Read the model definition and answer for the solid it produces. Units are mm, in the model's axes. A direction names the side the tool comes from. Round coordinates to 2 decimals unless told otherwise and drop trailing zeros. Write each loop counter-clockwise with the first axis right and the second up, starting at its lowest first coordinate (ties: lowest second). Pieces come first, ordered by that corner, then holes.
from build123d import *

# Parameters (mm, degrees)
SKETCH034_R     = 3.75
POCKET013_DEPTH = 9.70192
CHAMFER013_SIZE = 0.4
CHAMFER014_SIZE = 0.1


with BuildPart() as pocket013:
    # Sketch035 → Revolution005 (revolve)
    with BuildSketch(Plane.XZ):
        Polygon((0, 0.29908), (2.75, 1.3), (2.75, 10), (0, 10), align=None)
    revolve(axis=Axis((0, 0, 0), (0, 0, 1)))

    # Sketch034 (on Face3 of Revolution005) → Pocket013 (cut, through all)
    with BuildSketch(Plane(origin=(0, 0, 10), x_dir=(-1, 0, 0), z_dir=(0, 0, 1))):
        Circle(SKETCH034_R)
        Polygon((-0.721688, 1.25), (0.721688, 1.25), (1.443376, 0), (0.721688, -1.25), (-0.721688, -1.25), (-1.443376, 0), align=None, mode=Mode.SUBTRACT)
    extrude(amount=-POCKET013_DEPTH, mode=Mode.SUBTRACT)


with BuildPart() as chamfer014:
    # Sketch033 → Revolution004 (revolve)
    with BuildSketch(Plane.XZ):
        Polygon((1.45, 3), (2.75, 3), (2.75, 0), (1.5, 0), (1.5, -10), (0, -10), (0, 1.549999), align=None)
    revolve(axis=Axis((0, 0, 0), (0, 0, 1)))

    # Cut005: cut Pocket013
    add(pocket013.part, mode=Mode.SUBTRACT)

    # Chamfer013
    chamfer013_edges = [chamfer014.edges().sort_by_distance(p)[0] for p in [
        (-1.5, 0, -10),
    ]]
    chamfer(chamfer013_edges, length=CHAMFER013_SIZE)

    # Chamfer014
    chamfer014_edges = [chamfer014.edges().sort_by_distance(p)[0] for p in [
        (-2.75, 0, 0),
        (-2.75, 0, 3),
    ]]
    chamfer(chamfer014_edges, length=CHAMFER014_SIZE)


solid = chamfer014.part
Q1. Section A-A (z = 1.5) is taken. Determine the outline of the cut face in (x, y), then the cut area to 3 significant figures.
Verdict:
outline: circle Ø5.5 at (0, 0); hole (-1.44, 0) - (-0.72, -1.25) - (0.72, -1.25) - (1.44, 0) - (0.72, 1.25) - (-0.72, 1.25) - close
area: 18.3 mm2
Q2. Section B-B (z = -1.5) is taken. Determine the outline of the cut face in (x, y), then the cut area to 3 significant figures.
Verdict:
outline: circle Ø3 at (0, 0)
area: 7.07 mm2
Q3. Straight lines are drawn through the part: probe 1 along Z at (x, y) = (0.45, 1.75); probe 2 along Y at (x, z) = (-1.1, 1); probe 3 along Y at (x, z) = (-1.15, 2.5). For each, find the intervals that lie inside material, in ascending order.
Verdict:
probe 1: z = 0 to 3
probe 2: y = -2.52 to -0.59, 0.59 to 2.52
probe 3: y = -2.5 to -0.51, 0.51 to 2.5
Q4. A flat-ended cylindrical pin translates along its axis: pin 1 Ø1.5 at (x, z) = (2, -3.5) entering from -Y. Find the tip coordinate at first contact, or state that the pin passes through.
Verdict:
pin 1: stops at y = -0.83
Q5. Which of the six approach directions +Z, -Z, +X, -X, +Y, -Y give full straight-line access (tool end or side, diameter ignored) to faces 1 (the flat face through (0, -2, 0)), 2 (the flat face through (0, 0, -10)), 3 (the flat face through (1.088, -0.616, 1.889))?
Verdict:
face 1: -Z
face 2: -Z, +X, -X, +Y, -Y
face 3: +Z
